Input: part model. Units: mm. Frame: model coordinates. Face numbers are marked on the shaded views. A direction names the side the tool comes from. Give positions to 0.01 mm unless a question says otherwise; leave off trailing zeros. Write each loop counter-clockwise with the first axis right and the second up, starting at its lowest first coordinate (ties: lowest second). Pieces come first, ordered by that corner, then holes. Notation, with made-up numbers: (85.5, 52) - (99.5, 52) arc R12 ccw to (99.5, 59) - close; hole circle Ø5 at (32.25, 15.5). An arc over 180 degrees is marked (long way). Answer as CSV lines item,"result".
```python
from build123d import *

# Parameters (mm, degrees)
SKETCH_1_W          = 26
SKETCH_1_H          = 38
EXTRUDE_1_DEPTH     = 12
SKETCH_2_W          = 22
SKETCH_2_H          = 34
CUT_EXTRUDE_1_DEPTH = 10
SKETCH_3_W          = 2.25
SKETCH_3_H          = 7.25
CUT_EXTRUDE_3_DEPTH = 12
SKETCH_4_W          = 6
SKETCH_4_H          = 6
EXTRUDE_2_DEPTH     = 5
SKETCH_5_R          = 1.5
CUT_EXTRUDE_4_DEPTH = 13
CUT_EXTRUDE_START   = 2
CUT_EXTRUDE_5_DEPTH = 1.6
SKETCH_7_R          = 12
SKETCH_7_R_2        = 11
EXTRUDE_3_DEPTH     = 5
SKETCH_9_R          = 11
CUT_EXTRUDE_7_DEPTH = 1
SKETCH_10_W         = 14.41096837
SKETCH_10_H         = 3
EXTRUDE_4_DEPTH     = 2
CUT_EXTRUDE_START_2 = 20
SKETCH_11_W         = 2
SKETCH_11_H         = 4.5
CUT_EXTRUDE_8_DEPTH = 7
CUT_EXTRUDE_START_3 = -20
SKETCH_13_W         = 2
SKETCH_13_H         = 4.5
CUT_EXTRUDE_9_DEPTH = 7


with BuildPart() as part:
    # ｽｹｯﾁ1 → ﾎﾞｽ - 押し出し1 (new body)
    with BuildSketch(Plane.XY):
        Rectangle(SKETCH_1_W, SKETCH_1_H)
    extrude(amount=EXTRUDE_1_DEPTH)

    # ｽｹｯﾁ2 → ｶｯﾄ - 押し出し1 (cut)
    with BuildSketch(Plane.XY):
        Rectangle(SKETCH_2_W, SKETCH_2_H)
    extrude(amount=CUT_EXTRUDE_1_DEPTH, mode=Mode.SUBTRACT)

    # ｽｹｯﾁ3 → ｶｯﾄ - 押し出し3 (cut)
    with BuildSketch(Plane.XY):
        with Locations((0, 4.375)):
            Rectangle(SKETCH_3_W, SKETCH_3_H)
    extrude(amount=CUT_EXTRUDE_3_DEPTH, mode=Mode.SUBTRACT)

    # ｽｹｯﾁ4 → ﾎﾞｽ - 押し出し2 (add)
    with BuildSketch(Plane.XY):
        with Locations((16, 16)):
            Rectangle(SKETCH_4_W, SKETCH_4_H)
        with Locations((16, -16)):
            Rectangle(SKETCH_4_W, SKETCH_4_H)
        with Locations((-16, -16)):
            Rectangle(SKETCH_4_W, SKETCH_4_H)
        with Locations((-16, 16)):
            Rectangle(SKETCH_4_W, SKETCH_4_H)
    extrude(amount=EXTRUDE_2_DEPTH)

    # ｽｹｯﾁ5 → ｶｯﾄ - 押し出し4 (cut, through all)
    with BuildSketch(Plane.XY):
        with Locations((-16, 16)):
            Circle(SKETCH_5_R)
        with Locations((-16, -16)):
            Circle(SKETCH_5_R)
        with Locations((16, -16)):
            Circle(SKETCH_5_R)
        with Locations((16, 16)):
            Circle(SKETCH_5_R)
    extrude(amount=CUT_EXTRUDE_4_DEPTH, mode=Mode.SUBTRACT)

    # ｽｹｯﾁ6 → ｶｯﾄ - 押し出し5 (cut)
    with BuildSketch(Plane.XY.offset(CUT_EXTRUDE_START)):
        Polygon((-17.184124892, 17.98272075), (-18.309148984, 15.965878137), (-17.125024092, 13.983157387), (-14.815875108, 14.01727925), (-13.690851016, 16.034121863), (-14.874975908, 18.016842613), align=None)
        Polygon((-17.154700538, -14), (-18.309401077, -16), (-17.154700538, -18), (-14.845299462, -18), (-13.690598923, -16), (-14.845299462, -14), align=None)
        Polygon((14.845299462, 18), (13.690598923, 16), (14.845299462, 14), (17.154700538, 14), (18.309401077, 16), (17.154700538, 18), align=None)
        Polygon((14.854466591, -13.994735294), (13.690623119, -15.98942868), (14.836156527, -17.994693386), (17.145533409, -18.005264706), (18.309376881, -16.01057132), (17.163843473, -14.005306614), align=None)
    extrude(amount=CUT_EXTRUDE_5_DEPTH, mode=Mode.SUBTRACT)

    # ｽｹｯﾁ7 → ﾎﾞｽ - 押し出し3 (add)
    with BuildSketch(Plane.XY.offset(12)):
        with Locations((0, 7)):
            Circle(SKETCH_7_R)
        with Locations((0, 7)):
            Circle(SKETCH_7_R_2, mode=Mode.SUBTRACT)
    extrude(amount=EXTRUDE_3_DEPTH)

    # ｽｹｯﾁ9 → ｶｯﾄ - 押し出し7 (cut)
    with BuildSketch(Plane.XY.offset(12)):
        with Locations((0, 7)):
            Circle(SKETCH_9_R)
    extrude(amount=-CUT_EXTRUDE_7_DEPTH, mode=Mode.SUBTRACT)

    # ｽｹｯﾁ10 → ﾎﾞｽ - 押し出し4 (add)
    with BuildSketch(Plane.XY.offset(10)):
        with Locations((0, -11.5)):
            Rectangle(SKETCH_10_W, SKETCH_10_H)
    extrude(amount=-EXTRUDE_4_DEPTH)

    # ｽｹｯﾁ11 → ｶｯﾄ - 押し出し8 (cut)
    with BuildSketch(Plane(origin=(0, 0, 0), x_dir=(0, 0, -1), z_dir=(1, 0, 0)).offset(CUT_EXTRUDE_START_2)):
        with Locations((-3, 16)):
            Rectangle(SKETCH_11_W, SKETCH_11_H)
        with Locations((-3, -16)):
            Rectangle(SKETCH_11_W, SKETCH_11_H)
    extrude(amount=-CUT_EXTRUDE_8_DEPTH, mode=Mode.SUBTRACT)

    # ｽｹｯﾁ13 → ｶｯﾄ - 押し出し9 (cut)
    with BuildSketch(Plane(origin=(0, 0, 0), x_dir=(0, 0, -1), z_dir=(1, 0, 0)).offset(CUT_EXTRUDE_START_3)):
        with Locations((-3, 16)):
            Rectangle(SKETCH_13_W, SKETCH_13_H)
        with Locations((-3, -16)):
            Rectangle(SKETCH_13_W, SKETCH_13_H)
    extrude(amount=CUT_EXTRUDE_9_DEPTH, mode=Mode.SUBTRACT)


solid = part.part
```
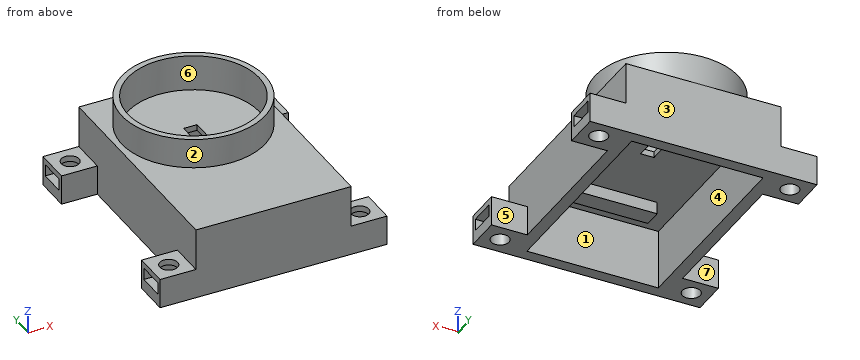
Item 1: Ray query, line 1 (Y direction, x = -16, z = 4.4); line 2 (X direction, y = 16, z = 4.3); line 3 (X direction, y = 0, z = 2). Return the intervals inside material, ascending. Write a range as from..to.
The answers:
line 1,"-19..-17.5, -14.5..-13, 13..14.5, 17.5..19"
line 2,"-19..-17.5, -14.5..-11, 11..14.5, 17.5..19"
line 3,"-13..-11, 11..13"
Item 2: Cut plane D-D on x = -3.5. Return the cut outline in (y, z).
The answers:
outline,"(-19, 0) - (-17, 0) - (-17, 10) - (-13, 10) - (-13, 8) - (-10, 8) - (-10, 10) - (17, 10) - (17, 0) - (19, 0) - (19, 12) - (18.48, 12) - (18.48, 17) - (17.43, 17) - (17.43, 11) - (-3.43, 11) - (-3.43, 17) - (-4.48, 17) - (-4.48, 12) - (-19, 12) - close"
Item 3: Cut plane B-B on x = 16. Count the separate pieces of the cut face and the enclosed holes in it, plus the area to 3 significant figures.
The answers:
separate pieces,"4"
enclosed holes,"0"
area,"24.0 mm²"
Item 4: Cut plane A-A on y = 7. Return the cut outline in (x, z) (3 decimals).
The answers:
outline,"(-13, 0) - (-11, 0) - (-11, 10) - (-1.125, 10) - (-1.125, 11) - (-11, 11) - (-11, 17) - (-12, 17) - (-12, 12) - (-13, 12) - close; (1.125, 10) - (11, 10) - (11, 0) - (13, 0) - (13, 12) - (12, 12) - (12, 17) - (11, 17) - (11, 11) - (1.125, 11) - close"
Item 5: Contact query for flat-ended pins moving along their axis: pin 1 (1 mm diameter, centred on y = -2, z = 14.5, fed in from -X); pin 2 (1.6 mm diameter, centred on y = -16, z = 3, fed in from +X); pin 3 (1 mm diameter, centred on y = 5, z = 3.5, fed in from -X). Output: stop coordinate, or through.
The answers:
pin 1,"x = -8.47"
pin 2,"x = 13"
pin 3,"x = -13"
Item 6: Reachability of the marked faces 4, 5, 6 and 7 from +Z, -Z, +X, -X, +Y, -Y: full face, straight path, thin tool, end or side. Return the list, or none.
The answers:
face 4,"-Z"
face 5,"+Z, -Z, +X"
face 6,"+Z"
face 7,"+Z, -Z, -X"
Item 7: Mould query, pull axis X, two halves, no side actions, for the marked faces 1, 2 and 3. Classes: +X half, -X half, draft (parallel to the pull), parting line (faces both ways), or undercut.
The answers:
face 1,"undercut"
face 2,"parting line"
face 3,"draft"
